Build history of the part. All positions in model axes, mm. Face numbers are marked on the shaded views. Coordinates: 2 decimals unless noted, no trailing zeros. Order: outer loops, then holes, each group sorted by start corner. A loop starts at its lowest first (then second) coordinate and runs counter-clockwise, first axis right, second up. Notation, with made-up numbers: (13.25, 13.5) - (61.25, 13.5) arc R30 ccw to (61.25, 41.5) - close; hole circle Ø11 at (42, 32). An arc over 180 degrees is marked (long way). Return JSON: item names as keys, results as strings.
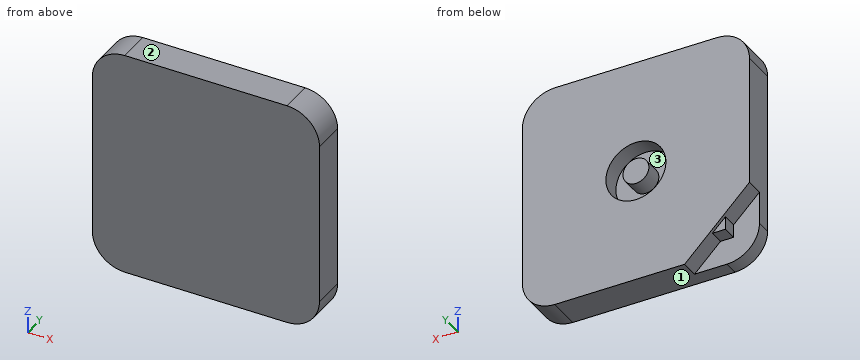
from build123d import *

# Parameters (mm, degrees)
SKETCH_1_W          = 70
SKETCH_1_H          = 70
EXTRUDE_1_DEPTH     = 10
SKETCH_2_R          = 9.25
CUT_EXTRUDE_1_DEPTH = 5.5
SKETCH_3_R          = 4
EXTRUDE_2_DEPTH     = 5.5
CUT_EXTRUDE_2_DEPTH = 5.5
EXTRUDE_3_DEPTH     = 4.5
FILLET_1_R          = 10


with BuildPart() as part:
    # 草图1 → 凸台-拉伸1 (new body)
    with BuildSketch(Plane(origin=(0, 0, 0), x_dir=(1, 0, 0), z_dir=(0, 1, 0))):
        Rectangle(SKETCH_1_W, SKETCH_1_H)
    extrude(amount=EXTRUDE_1_DEPTH)

    # 草图2 → 切除-拉伸1 (cut)
    with BuildSketch(Plane(origin=(0, 10, 0), x_dir=(1, 0, 0), z_dir=(0, 1, 0))):
        Circle(SKETCH_2_R)
    extrude(amount=-CUT_EXTRUDE_1_DEPTH, mode=Mode.SUBTRACT)

    # 草图3 → 凸台-拉伸2 (add)
    with BuildSketch(Plane(origin=(0, 4.5, 0), x_dir=(1, 0, 0), z_dir=(0, 1, 0))):
        Circle(SKETCH_3_R)
    extrude(amount=EXTRUDE_2_DEPTH)

    # 草图4 → 切除-拉伸2 (cut)
    with BuildSketch(Plane(origin=(0, 10, 0), x_dir=(1, 0, 0), z_dir=(0, 1, 0))):
        Polygon((-35, 35), (-15, 35), (-35, 15), align=None)
    extrude(amount=-CUT_EXTRUDE_2_DEPTH, mode=Mode.SUBTRACT)

    # 草图5 → 凸台-拉伸3 (add)
    with BuildSketch(Plane(origin=(0, 4.5, 0), x_dir=(1, 0, 0), z_dir=(0, 1, 0))):
        Polygon((-23, 27), (-27, 27), (-27, 23), align=None)
    extrude(amount=EXTRUDE_3_DEPTH)

    # 圆角1
    fillet_1_edges = [part.edges().sort_by_distance(p)[0] for p in [
        (-35, 2.25, -35),
        (35, 5, 35),
        (-35, 5, 35),
        (35, 5, -35),
    ]]
    fillet(fillet_1_edges, radius=FILLET_1_R)


solid = part.part
1. Cut at B-B on x = 0. Give the cut face in (y, z).
Check values:
{"outline": "(0, -35) - (10, -35) - (10, -9.25) - (4.5, -9.25) - (4.5, -4) - (10, -4) - (10, 4) - (4.5, 4) - (4.5, 9.25) - (10, 9.25) - (10, 35) - (0, 35) - close"}
2. Cut at A-A on y = 3.5. Give the cut face in (x, z).
Check values:
{"outline": "(-35, -25) arc R10 ccw to (-25, -35) - (25, -35) arc R10 ccw to (35, -25) - (35, 25) arc R10 ccw to (25, 35) - (-25, 35) arc R10 ccw to (-35, 25) - close"}
3. Drop a flat-ended pin along its axis: pin 1 (2 mm diameter, centred on x = -25, y = 7, fed in from -Z). Give the stop position or say it passes through.
Check values:
{"pin 1": "z = -27"}
4. Mould opens along Z. For the marked faces 1, 2 and 3 say: pulls with the +Z half, pulls with the -Z half, needs draft (parallel to the pull), parting line crosses it, or undercut.
Check values:
{"face 1": "pulls with the -Z half", "face 2": "pulls with the +Z half", "face 3": "undercut"}
5. Cut at D-D on x = -26. Give the cut face in (y, z).
Check values:
{"outline": "(0, -34.95) - (4.5, -34.95) - (4.5, -27) - (9, -27) - (9, -24) - (10, -24) - (10, 34.95) - (0, 34.95) - close"}
6. Cut at C-C on z = 0. Give the cut face in (x, y), plus the area to 3 significant figures.
Check values:
{"outline": "(-35, 0) - (35, 0) - (35, 10) - (9.25, 10) - (9.25, 4.5) - (4, 4.5) - (4, 10) - (-4, 10) - (-4, 4.5) - (-9.25, 4.5) - (-9.25, 10) - (-35, 10) - close", "area": "642 mm²"}
7. Probe L1, parallel to X at y = 6.2, z = 0; L2, parallel to X at y = 7, z = -2.5. List the from-to ranges inside material, lowest first.
Check values:
{"L1": "-35 to -9.25, -4 to 4, 9.25 to 35", "L2": "-35 to -8.91, -3.12 to 3.12, 8.91 to 35"}
